```python
from build123d import *

# Parameters (mm, degrees)
F0_W     = 31.496
F0_H     = 15.621
F1_DEPTH = 9.1948
F3_R     = 2.79439
F4_DEPTH = 2.032
F5_W     = 28.9306
F5_H     = 13.208
F6_DEPTH = 8.6614
F7_R     = 3.0861
F8_DEPTH = 8.6614


with BuildPart() as f1:
    # F0 (on Top) → F1 (new body)
    with BuildSketch(Plane.XY):
        Rectangle(F0_W, F0_H)
    extrude(amount=F1_DEPTH)

    # F3 (on offset) → F4 (join)
    with BuildSketch(Plane.XY.offset(9.1948)):
        with Locations((-11.9507, 3.9624)):
            Circle(F3_R)
        with Locations((-3.9751, 3.9624)):
            Circle(F3_R)
        with Locations((4.0005, 3.9624)):
            Circle(F3_R)
        with Locations((11.9761, 3.9624)):
            Circle(F3_R)
        with Locations((-11.9507, -4.08486)):
            Circle(F3_R)
        with Locations((-3.9751, -4.08486)):
            Circle(F3_R)
        with Locations((4.0005, -4.08486)):
            Circle(F3_R)
        with Locations((11.9761, -4.08486)):
            Circle(F3_R)
    extrude(amount=F4_DEPTH)

    # F5 (on Top) → F6 (cut)
    with BuildSketch(Plane.XY):
        Rectangle(F5_W, F5_H)
    extrude(amount=F6_DEPTH, mode=Mode.SUBTRACT)

    # F7 (on Top) → F8 (join)
    with BuildSketch(Plane.XY):
        Circle(F7_R)
        with Locations((8.7122, 0)):
            Circle(F7_R)
        with Locations((-8.7122, 0)):
            Circle(F7_R)
    extrude(amount=F8_DEPTH)


solid = f1.part
```
Input: part model. Units: mm. Frame: model coordinates. A direction names the side the tool comes from. Give positions to 0.01 mm unless a question says otherwise; leave off trailing zeros. Order: outer loops, then holes, each group sorted by start corner. A loop starts at its lowest first (then second) coordinate and runs counter-clockwise, first axis right, second up.
1. Section B-B on x = 0. Return the cut outline in (y, z).
Derived:
outline: (-7.81, 0) - (-6.6, 0) - (-6.6, 8.66) - (-3.09, 8.66) - (-3.09, 0) - (3.09, 0) - (3.09, 8.66) - (6.6, 8.66) - (6.6, 0) - (7.81, 0) - (7.81, 9.19) - (-7.81, 9.19) - close
2. Section D-D on z = 10. Return the cut outline in (x, y), and give its area (3 significant figures).
Derived:
outline: circle Ø5.59 at (-11.95, -4.08); circle Ø5.59 at (-11.95, 3.96); circle Ø5.59 at (-3.98, -4.08); circle Ø5.59 at (-3.98, 3.96); circle Ø5.59 at (4, -4.08); circle Ø5.59 at (4, 3.96); circle Ø5.59 at (11.98, -4.08); circle Ø5.59 at (11.98, 3.96)
area: 196 mm2
3. Section A-A on z = 4.75. Return the cut outline in (x, y).
Derived:
outline: (-15.75, -7.81) - (15.75, -7.81) - (15.75, 7.81) - (-15.75, 7.81) - close; circle Ø6.17 at (-8.71, 0); circle Ø6.17 at (0, 0); circle Ø6.17 at (8.71, 0); hole (-14.47, -6.6) - (14.47, -6.6) - (14.47, 6.6) - (-14.47, 6.6) - close
4. Material intervals for L1, parallel to X at y = 5.5, z = 3; L2, parallel to Y at x = 7, z = 5.5; L3, parallel to X at y = 2, z = 7.5, sorted ascending.
Derived:
L1: x = -15.75 to -14.47, 14.47 to 15.75
L2: y = -7.81 to -6.6, -2.57 to 2.57, 6.6 to 7.81
L3: x = -15.75 to -14.47, -11.06 to -6.36, -2.35 to 2.35, 6.36 to 11.06, 14.47 to 15.75
5. Mould query, pull axis Y, two halves, no side actions, for faces 4 (the cylindrical face through (-11.16, -1.88, 4.27)), 5 (the flat face through (0, -7.81, 5)), 6 (the flat face through (-12, -4, 11.227)). Classes: released by +Y, released by -Y, zero draft, split by the parting line, or undercut.
Derived:
face 4: undercut
face 5: released by -Y
face 6: zero draft
6. Section C-C on y = 0. Return the cut outline in (x, z), and give its area (3 significant figures).
Derived:
outline: (-15.75, 0) - (-14.47, 0) - (-14.47, 8.66) - (-11.8, 8.66) - (-11.8, 0) - (-5.63, 0) - (-5.63, 8.66) - (-3.09, 8.66) - (-3.09, 0) - (3.09, 0) - (3.09, 8.66) - (5.63, 8.66) - (5.63, 0) - (11.8, 0) - (11.8, 8.66) - (14.47, 8.66) - (14.47, 0) - (15.75, 0) - (15.75, 9.19) - (-15.75, 9.19) - close
area: 199 mm2
7. Reachability of faces 1 (the cylindrical face through (-2.686, -6.564, 10.197)), 2 (the cylindrical face through (11.656, 0.927, 4.27)), 3 (the flat face through (4, -4, 11.227)) from +Z, -Z, +X, -X, +Y, -Y: full face, straight path, thin tool, end or side. Return the list, or none.
Derived:
face 1: +Z
face 2: -Z
face 3: +Z, +X, -X, +Y, -Y
8. Pin query (flat end, axial travel): pin 1 (8 mm diameter, centred on x = -0.5, y = 1, fed in from +Z). Return the tip coordinate at first contact, or that it passes through.
Derived:
pin 1: stops at z = 11.23
